Drawing for the job (mm, zero at the part's lowest x, y, z). A direction names the side the tool comes from. Give positions to 0.01 mm unless a question says otherwise; leave off trailing zeros. Loops run counter-clockwise (first coordinate to the right, second up) from the corner with the lowest first, then second, coordinate; pieces in that order, holes last. Notation, with made-up numbers: (50, 25) -> (63, 25) arc R20 cw to (63, 59) -> close; hole circle Ø1 at (85.5, 80.25). An arc over 180 degrees is marked (long way). Write item = value, one per line.
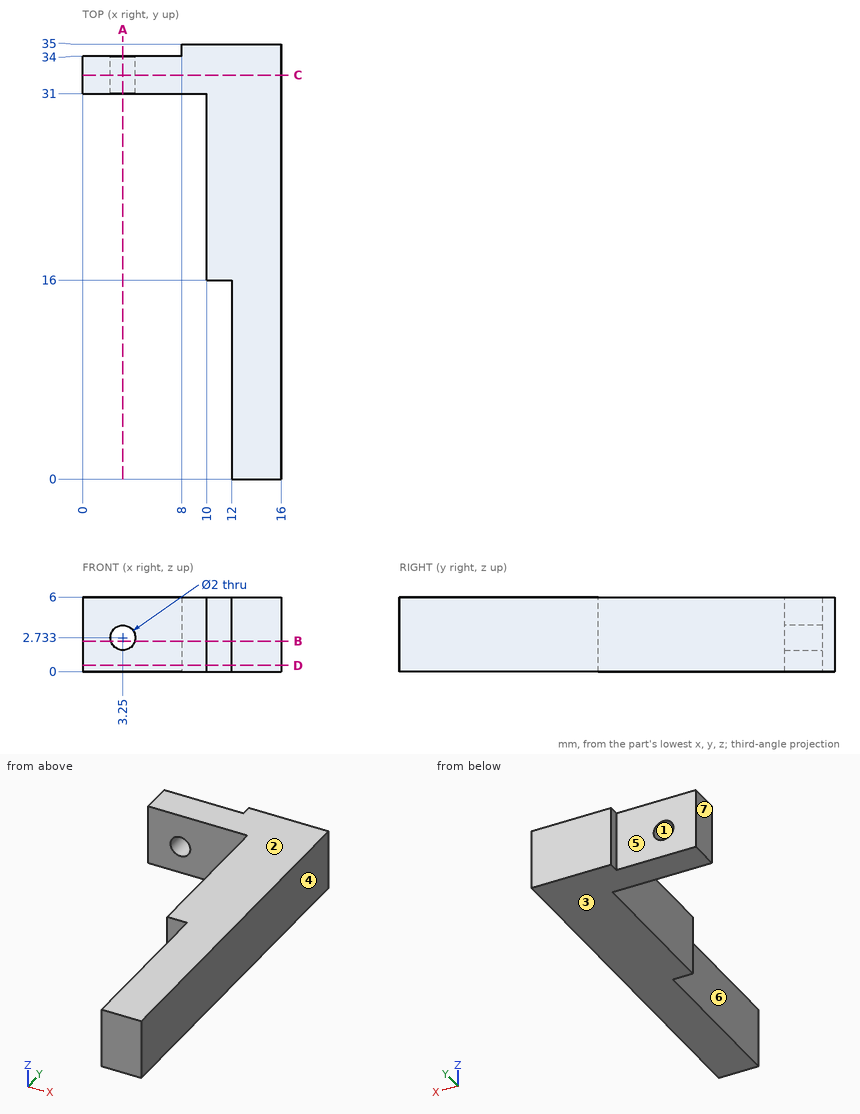
1) Slice it at D-D, the plane z = 0.5. List the corners of the cut face in (x, y), and give its area (3 significant figures).
Resolved:
outline = (0, 31) -> (10, 31) -> (10, 16) -> (12, 16) -> (12, 0) -> (16, 0) -> (16, 35) -> (8, 35) -> (8, 34) -> (0, 34) -> close
area = 210 mm²
2) Drill centre lines: line 1 along Y through (x, z) = (11.5, 0.7); line 2 along X through (y, z) = (12, 0.95); line 3 along X through (y, z) = (19.5, 3.25). Where is each one in solid material? Low to high. Write a range as [from, to].
Resolved:
line_1 = [16, 35]
line_2 = [12, 16]
line_3 = [10, 16]
3) Slice it at A-A, the plane x = 3.25. List the corners of the cut face in (y, z), and give its area (3 significant figures).
Resolved:
outline = (31, 0) -> (34, 0) -> (34, 1.73) -> (31, 1.73) -> close; (31, 3.73) -> (34, 3.73) -> (34, 6) -> (31, 6) -> close
area = 12.0 mm²
4) Slice it at B-B, the plane z = 2.45. List the corners of the cut face in (x, y).
Resolved:
outline = (0, 31) -> (2.29, 31) -> (2.29, 34) -> (0, 34) -> close; (4.21, 31) -> (10, 31) -> (10, 16) -> (12, 16) -> (12, 0) -> (16, 0) -> (16, 35) -> (8, 35) -> (8, 34) -> (4.21, 34) -> close
5) Which spindle directions (+Z, -Z, +X, -X, +Y, -Y) get a long thin tool onto all of the face, cutting with end or side? Do the marked faces 5, 6 and 7. Say none if no direction does.
Resolved:
face_5 = +Z, -Z, -X, +Y
face_6 = +Z, -Z, -X, -Y
face_7 = +Z, -Z, -X, +Y, -Y
6) Pull direction Z, two halves, no side cores. Call the marked faces 1, 2, 3 and 4: pulls with the +Z half, pulls with the -Z half, needs draft (parallel to the pull), parting line crosses it, or undercut.
Resolved:
face_1 = undercut
face_2 = pulls with the +Z half
face_3 = pulls with the -Z half
face_4 = needs draft
7) Slice it at C-C, the plane y = 32.5. List the corners of the cut face in (x, z).
Resolved:
outline = (0, 0) -> (16, 0) -> (16, 6) -> (0, 6) -> close; hole circle Ø2 at (3.25, 2.73)
8) Drop flat-ended pins along their axis: P1, Ø2, axis at x = 2, z = 5, coming from the +Y side; P2, Ø3, axis at y = 9.5, z = 1, coming from the -X side; P3, Ø1.8, axis at x = 3.25, z = 2.73, coming from the -Y side; P4, Ø1.5, axis at y = 22, z = 5, coming from the -X side. Give the stop position or say it passes through.
Resolved:
P1 = 34
P2 = 12
P3 = through
P4 = 10
